Can you work these out from the model? Positions are in its coordinate system, mm. A direction names the side the tool comes from. Give positions to 0.01 mm unless a question says otherwise; leave off trailing zeros. Write each loop counter-clockwise with the first axis right and the second up, starting at its lowest first coordinate (ties: lowest second). Pieces come first, ordered by that corner, then holes.
from build123d import *

# Parameters (mm, degrees)
SKETCH_W      = 28
SKETCH_H      = 39
SKETCH_W_2    = 25
SKETCH_H_2    = 32
PAD_DEPTH     = 40
SKETCH001_W   = 28
SKETCH001_H   = 39
SKETCH001_W_2 = 15
SKETCH001_H_2 = 5
PAD001_DEPTH  = 2


with BuildPart() as part:
    # Sketch → Pad (new body)
    with BuildSketch(Plane.XY):
        with Locations((14, 19.5)):
            Rectangle(SKETCH_W, SKETCH_H)
        with Locations((14, 19.5)):
            Rectangle(SKETCH_W_2, SKETCH_H_2, mode=Mode.SUBTRACT)
    extrude(amount=PAD_DEPTH)

    # Sketch001 (on Face9 of Pad) → Pad001 (join)
    with BuildSketch(Plane(origin=(0, 0, 0), x_dir=(1, 0, 0), z_dir=(0, 0, -1))):
        with Locations((14, -19.5)):
            Rectangle(SKETCH001_W, SKETCH001_H)
        with Locations((14, -7.5)):
            Rectangle(SKETCH001_W_2, SKETCH001_H_2, mode=Mode.SUBTRACT)
    extrude(amount=PAD001_DEPTH)


solid = part.part
(1) Will this pin go through, and if not, where does the flat tip stop? P1, Ø4, axis at x = 18.5, y = 14, coming from the +Z side.
Returned:
P1: stops at z = 0
(2) Imagine slicing it at C-C, the plane z = 26.5. Write out the boundary of the cut face in (x, y), plus the area to 3 significant figures.
Returned:
outline: (0, 0) - (28, 0) - (28, 39) - (0, 39) - close; hole (1.5, 3.5) - (26.5, 3.5) - (26.5, 35.5) - (1.5, 35.5) - close
area: 292 mm2
(3) For faces 1 (the face through (14, 3.5, 20)), 2 (the face through (21.5, 8, -1)), 3 (the face through (14, 19, -2)), which set-ups out of +Z, -Z, +X, -X, +Y, -Y let a thin tool reach every point of the face, with its end or its side?
Returned:
face 1: +Z
face 2: +Z, -Z
face 3: -Z, +X, -X, +Y, -Y
(4) Imagine slicing it at A-A, the plane y = 9. Write out the boundary of the cut face in (x, z), plus the area to 3 significant figures.
Returned:
outline: (0, -2) - (6.5, -2) - (6.5, 0) - (1.5, 0) - (1.5, 40) - (0, 40) - close; (21.5, -2) - (28, -2) - (28, 40) - (26.5, 40) - (26.5, 0) - (21.5, 0) - close
area: 146 mm2
(5) If I drill on L1, parallel to X at y = 17, z = 20.5; L2, parallel to Y at x = 21, z = 23; L3, parallel to Z at x = 8.75, y = 28, over which ranges is the centre line in solid material (lowest first)?
Returned:
L1: x = 0 to 1.5, 26.5 to 28
L2: y = 0 to 3.5, 35.5 to 39
L3: z = -2 to 0
(6) Imagine slicing it at D-D, the plane y = 14. Write out the boundary of the cut face in (x, z), plus the area to 3 significant figures.
Returned:
outline: (0, -2) - (28, -2) - (28, 40) - (26.5, 40) - (26.5, 0) - (1.5, 0) - (1.5, 40) - (0, 40) - close
area: 176 mm2
(7) If we mould it in two halves opening along X, with no side actions, what happens to faces 4 (the face through (14, 39, 19)), 5 (the face through (28, 20, 19)), 6 (the face through (0, 20, 19)), 7 (the face through (6.5, 8, -1))? For each: +X half, -X half, draft (parallel to the pull), parting line (faces both ways), or undercut.
Returned:
face 4: draft
face 5: +X half
face 6: -X half
face 7: undercut
(8) Imagine slicing it at B-B, the plane x = 20.75. Write out the boundary of the cut face in (y, z).
Returned:
outline: (0, -2) - (5, -2) - (5, 0) - (3.5, 0) - (3.5, 40) - (0, 40) - close; (10, -2) - (39, -2) - (39, 40) - (35.5, 40) - (35.5, 0) - (10, 0) - close
